```python
from build123d import *

# Parameters (mm, degrees)
SKETCH_2_R          = 6.5
EXTRUDE_1_DEPTH     = 2
SKETCH_3_R          = 2
CUT_EXTRUDE_2_DEPTH = 10.407443861
EXTRUDE_START       = -2
EXTRUDE_2_DEPTH     = 2
EXTRUDE_3_DEPTH     = 2
SKETCH_22_R         = 9
SKETCH_22_R_2       = 1
CUT_EXTRUDE_4_DEPTH = 2
CHAMFER_1_SIZE      = 2


with BuildPart() as part:
    # 草图2 → 凸台-拉伸1 (new body)
    with BuildSketch(Plane(origin=(0, 0, 0), x_dir=(1, 0, 0), z_dir=(0, 1, 0))):
        with Locations(Location((0, 0, 0), (0, 0, 270))):
            Circle(SKETCH_2_R)
    extrude(amount=EXTRUDE_1_DEPTH)

    # 草图3 → 切除-拉伸2 (cut, through all)
    with BuildSketch(Plane(origin=(0, 2, 0), x_dir=(1, 0, 0), z_dir=(0, 1, 0))):
        with Locations(Location((0, 0, 0), (0, 0, 270))):
            Circle(SKETCH_3_R)
    extrude(amount=-CUT_EXTRUDE_2_DEPTH, mode=Mode.SUBTRACT)

    # 草图4 → 凸台-拉伸2 (add)
    with BuildSketch(Plane(origin=(0, 2, 0), x_dir=(1, 0, 0), z_dir=(0, 1, 0)).offset(EXTRUDE_START)):
        with BuildLine():
            Line((6.5, 0), (6.5, 31))
            Line((6.5, 31), (3.899148682, 31))
            Line((3.899148682, 31), (-4.100851318, 31))
            Line((-4.100851318, 31), (-6.5, 31))
            Line((-6.5, 31), (-6.5, 0))
            ThreePointArc((-6.5, 0), (0, 6.5), (6.5, 0))
        make_face()
    extrude(amount=EXTRUDE_2_DEPTH)

    # 草图21 → 凸台-拉伸3 (add)
    with BuildSketch(Plane(origin=(0, 0, -31), x_dir=(-1, 0, 0), z_dir=(0, 0, -1))):
        Polygon((0, 0), (12, 0), (12, 25), (-12, 25), (-12, 0), align=None)
    extrude(amount=EXTRUDE_3_DEPTH)

    # 草图22 → 切除-拉伸4 (cut)
    with BuildSketch(Plane.XY.offset(-31)):
        with Locations((0, 13.5)):
            Circle(SKETCH_22_R)
        with Locations((7.7, 22.2)):
            Circle(SKETCH_22_R_2)
        with Locations((-7.7, 22.2)):
            Circle(SKETCH_22_R_2)
        with Locations((-7.7, 6.8)):
            Circle(SKETCH_22_R_2)
        with Locations((7.7, 6.8)):
            Circle(SKETCH_22_R_2)
    extrude(amount=-CUT_EXTRUDE_4_DEPTH, mode=Mode.SUBTRACT)

    # 倒角1
    chamfer_1_edges = [part.edges().sort_by_distance(p)[0] for p in [
        (12, 0, -32),
        (-12, 0, -32),
        (-12, 25, -32),
        (12, 25, -32),
    ]]
    chamfer(chamfer_1_edges, length=CHAMFER_1_SIZE)


solid = part.part
```
Geometry: final body of the model. Coordinates: model frame, mm. A direction names the side the tool comes from. Give positions to 0.01 mm unless a question says otherwise; leave off trailing zeros. Loops run counter-clockwise (first coordinate to the right, second up) from the corner with the lowest first, then second, coordinate; pieces in that order, holes last. Notation, with made-up numbers: (79, 3.5) -> (120, 3.5) arc R21 cw to (120, 22.5) -> close; hole circle Ø8 at (7, 38.5). An arc over 180 degrees is marked (long way). Return JSON: item names as keys, results as strings.
Item 1: Pin query (flat end, axial travel): P1, Ø1.5, axis at x = -8, z = -15, coming from the -Y side; P2, Ø1.6, axis at y = 1, z = -17, coming from the -X side; P3, Ø1, axis at y = 1, z = -9.5, coming from the +X side; P4, Ø4, axis at x = -1.5, z = -21, coming from the +Y side. Return the tip coordinate at first contact, or that it passes through.
Filled in:
{"P1": "through", "P2": "x = -6.5", "P3": "x = 6.5", "P4": "y = 2"}
Item 2: Mould query, pull axis Y, two halves, no side actions, for faces 4 (the flat face through (6, 21, -31)), 5 (the flat face through (11, 1, -32)), 6 (the cylindrical face through (-6.746, 7.1, -31.986)). Classes: released by +Y, released by -Y, zero draft, split by the parting line, or undercut.
Filled in:
{"face 4": "zero draft", "face 5": "released by -Y", "face 6": "undercut"}
Item 3: Access query for faces 1 (the flat face through (-11, 1, -32)), 2 (the flat face through (6.5, 1, -15)), 3 (the flat face through (0, 2, -13)). Directions: +Z, -Z, +X, -X, +Y, -Y. A direction counts if a zero-diameter tool reaches every point of the face in a straight line with its end or side. Return the directions, or none.
Filled in:
{"face 1": "+Z, -Z, -X, -Y", "face 2": "+Z, +X, +Y, -Y", "face 3": "+Z, +X, -X, +Y"}
Item 4: Section D-D, the plane y = 4. Output: boundary loops of the cut face in (x, z), plus the area to 3 significant figures.
Filled in:
{"outline": "(-12, -33) -> (12, -33) -> (12, -31) -> (-12, -31) -> close", "area": "48.0 mm^2"}
Item 5: Section A-A, the plane x = 0. Output: boundary loops of the cut face in (y, z), plus the area to 3 significant figures.
Filled in:
{"outline": "(0, -33) -> (4.5, -33) -> (4.5, -31) -> (2, -31) -> (2, -2) -> (0, -2) -> close; (0, 2) -> (2, 2) -> (2, 6.5) -> (0, 6.5) -> close; (22.5, -33) -> (25, -33) -> (25, -31) -> (22.5, -31) -> close", "area": "81.0 mm^2"}
Item 6: Section C-C, the plane y = 6.8. Output: boundary loops of the cut face in (x, z).
Filled in:
{"outline": "(-12, -33) -> (-8.7, -33) -> (-8.7, -31) -> (-12, -31) -> close; (-6.7, -33) -> (-6.01, -33) -> (-6.01, -31) -> (-6.7, -31) -> close; (6.01, -33) -> (6.7, -33) -> (6.7, -31) -> (6.01, -31) -> close; (8.7, -33) -> (12, -33) -> (12, -31) -> (8.7, -31) -> close"}
Item 7: Line query: line 1 (X direction, y = 1.65, z = 0); line 2 (Y direction, x = 0, z = -31.85); line 3 (Y direction, x = 2.25, z = -25.5). Output: solid intervals per line, ascending.
Filled in:
{"line 1": "-6.5 to -2, 2 to 6.5", "line 2": "0 to 4.5, 22.5 to 25", "line 3": "0 to 2"}
Item 8: Section B-B, the plane x = 7.7. Output: boundary loops of the cut face in (y, z), plus the area to 3 significant figures.
Filled in:
{"outline": "(0, -33) -> (5.8, -33) -> (5.8, -31) -> (0, -31) -> close; (7.8, -33) -> (8.84, -33) -> (8.84, -31) -> (7.8, -31) -> close; (18.16, -33) -> (21.2, -33) -> (21.2, -31) -> (18.16, -31) -> close; (23.2, -33) -> (25, -33) -> (25, -31) -> (23.2, -31) -> close", "area": "23.4 mm^2"}
